from build123d import *

# Parameters (mm, degrees)
SKETCH1_R               = 7.5
BOSS_EXTRUDE2_DEPTH     = 25
CUT_EXTRUDE1_DEPTH      = 24
CUT_EXTRUDE2_DEPTH      = 27
CUT_EXTRUDE2_DEPTH_BACK = 36
SKETCH3_R               = 0.4
SKETCH4_R               = 7
BOSS_EXTRUDE3_DEPTH     = 1
CUT_EXTRUDE3_START      = -11
SKETCH5_R               = 0.4
CUT_EXTRUDE3_DEPTH      = 11


with BuildPart() as part:
    # Sketch1 → Boss-Extrude2 (new body)
    with BuildSketch(Plane.XY):
        with BuildLine():
            ThreePointArc((2.414315168, 0.069999392), (0.769305306, 0.218548989), (-0.013240201, 1.673109733))
            Line((-0.013240201, 1.673109733), (-0.013240201, 23.326890267))
            ThreePointArc((-0.013240201, 23.326890267), (0.497304642, 24.55945455), (1.729868925, 25.069999392))
            Line((1.729868925, 25.069999392), (48.270131075, 25.069999392))
            ThreePointArc((48.270131075, 25.069999392), (49.605427649, 24.447342177), (49.986759799, 23.02421016))
            Line((49.986759799, 23.02421016), (49.986759799, 1.97578984))
            ThreePointArc((49.986759799, 1.97578984), (49.353809753, 0.307800264), (47.585684832, 0.069999392))
            Line((47.585684832, 0.069999392), (2.414315168, 0.069999392))
        make_face()
        with Locations((14.486759799, 15.569999392)):
            Circle(SKETCH1_R, mode=Mode.SUBTRACT)
        with Locations((35.513240201, 15.569999392)):
            Circle(SKETCH1_R, mode=Mode.SUBTRACT)
    extrude(amount=-BOSS_EXTRUDE2_DEPTH)

    # Sketch2 → Cut-Extrude1 (cut)
    with BuildSketch(Plane(origin=(0, 0, -25), x_dir=(-1, 0, 0), z_dir=(0, 0, -1))):
        with BuildLine():
            Line((-0.986759799, 1.673109733), (-0.986759799, 23.326890267))
            ThreePointArc((-0.986759799, 23.326890267), (-1.204411423, 23.852347769), (-1.729868925, 24.069999392))
            Line((-1.729868925, 24.069999392), (-48.270131075, 24.069999392))
            ThreePointArc((-48.270131075, 24.069999392), (-48.861025261, 23.777506771), (-48.986759799, 23.130282932))
            Line((-48.986759799, 23.130282932), (-48.986759799, 1.869717068))
            ThreePointArc((-48.986759799, 1.869717068), (-48.694204694, 1.062886218), (-47.836000807, 1.069999392))
            Line((-47.836000807, 1.069999392), (-2.163999193, 1.069999392))
            ThreePointArc((-2.163999193, 1.069999392), (-1.391043742, 1.011740949), (-0.986759799, 1.673109733))
        make_face()
    extrude(amount=-CUT_EXTRUDE1_DEPTH, mode=Mode.SUBTRACT)

    # Sketch3 → Cut-Extrude2 (cut, two sides: drawn at the far end of the back side and taken through both)
    with BuildSketch(Plane.XZ.offset(-0.069999392).offset(-CUT_EXTRUDE2_DEPTH_BACK)):
        with Locations(Location((25, -12.5, 0), (0, 0, 180))):
            Circle(SKETCH3_R)
    extrude(amount=CUT_EXTRUDE2_DEPTH + CUT_EXTRUDE2_DEPTH_BACK, mode=Mode.SUBTRACT)

    # Sketch4 → Boss-Extrude3 (add)
    with BuildSketch(Plane.XZ.offset(-0.069999392)):
        with Locations((25, -12.5)):
            Circle(SKETCH4_R)
    extrude(amount=BOSS_EXTRUDE3_DEPTH)

    # Sketch5 → Cut-Extrude3 (cut)
    with BuildSketch(Plane(origin=(0, 1.069999392, 0), x_dir=(1, 0, 0), z_dir=(0, 1, 0)).offset(CUT_EXTRUDE3_START)):
        with Locations(Location((25, 12.5, 0), (0, 0, 180))):
            Circle(SKETCH5_R)
    extrude(amount=CUT_EXTRUDE3_DEPTH, mode=Mode.SUBTRACT)


solid = part.part
Read the model definition and answer for the solid it produces. Units are mm, in the model's axes. A direction names the side the tool comes from. Round coordinates to 2 decimals unless told otherwise and drop trailing zeros. Write each loop counter-clockwise with the first axis right and the second up, starting at its lowest first coordinate (ties: lowest second). Pieces come first, ordered by that corner, then holes. Notation, with made-up numbers: (67.25, 58.25) - (121.25, 58.25) arc R10 ccw to (121.25, 71.25) - close; hole circle Ø2 at (-7, 51). An arc over 180 degrees is marked (long way). One line per question, with ' | ' between items. Start each with the question number.
1. Each of these flat-tipped pins is pushed along its axis until it touches: pin 1 (3 mm diameter, centred on x = 44.5, y = 8.5, fed in from -Z); pin 2 (10.5 mm diameter, centred on y = 17.5, z = -7, fed in from +X); pin 3 (2 mm diameter, centred on x = 18, z = -19.5, fed in from -Y); pin 4 (10 mm diameter, centred on x = 34.5, z = -18.5, fed in from -Y). Where does it stop, or does it pass through?
2. Section C-C (x = 33) is taken. Determine the outline of the cut face in (y, z).
3. Find the intervals of material crossed by probe 1 along X at (y, z) = (15.57, -0.45); probe 2 along X at (y, z) = (3.5, -3.5); probe 3 along Y at (x, z) = (12.5, -21.25), in increasing order. Write a range as [from, to].
4. For faces 5 (the face through (0.8, 0.2, -12.3)), 6 (the face through (48.705, 1.07, -13.168)), determine the directions among +Z, -Z, +X, -X, +Y, -Y from which every point of the face is accessible in a straight line to the end or side of a thin tool.
5. Section B-B (y = 10.5) is taken. Determine the outline of the cut face in (x, z).
6. For a pull along X with two mould halves and no side action, classify faces 1 (the face through (-0.013, 12, -12)), 2 (the face through (49.987, 13, -12)), 3 (the face through (24.7, 24.07, -13.2)), 4 (the face through (32.5, 0.5, -25)) as +X half, -X half, draft (parallel to the pull), parting line (faces both ways), or undercut.
7. Section D-D (y = 6.25) is taken. Determine the outline of the cut face in (x, z).
8. Section A-A (z = -22) is taken. Determine the outline of the cut face in (x, y), and give its area (3 significant figures).
Filled in:
1) pin 1: z = -1 | pin 2: x = 49.99 | pin 3: y = 0.07 | pin 4: y = -0.93
2) outline: (0.07, -25) - (1.07, -25) - (1.07, -1) - (8.5, -1) - (8.5, 0) - (0.07, 0) - close; (22.64, -1) - (24.07, -1) - (24.07, -25) - (25.07, -25) - (25.07, 0) - (22.64, 0) - close
3) probe 1: [-0.01, 6.99], [21.99, 28.01], [43.01, 49.99] | probe 2: [-0.01, 0.99], [48.99, 49.99] | probe 3: [0.07, 1.07], [24.07, 25.07]
4) face 5: +Z, -Z, -Y | face 6: -Z
5) outline: (-0.01, -25) - (0.99, -25) - (0.99, -1) - (8.96, -1) - (8.96, 0) - (-0.01, 0) - close; (20.01, -1) - (29.99, -1) - (29.99, 0) - (20.01, 0) - close; (41.04, -1) - (48.99, -1) - (48.99, -25) - (49.99, -25) - (49.99, 0) - (41.04, 0) - close
6) face 1: -X half | face 2: +X half | face 3: undercut | face 4: draft
7) outline: (-0.01, -25) - (0.99, -25) - (0.99, -1) - (48.99, -1) - (48.99, -25) - (49.99, -25) - (49.99, 0) - (-0.01, 0) - close
8) outline: (-0.01, 1.67) arc R1.74 ccw to (2.41, 0.07) - (47.59, 0.07) arc R1.74 ccw to (49.99, 1.98) - (49.99, 23.02) arc R1.74 ccw to (48.27, 25.07) - (1.73, 25.07) arc R1.74 ccw to (-0.01, 23.33) - close; hole (0.99, 1.67) arc R0.74 ccw to (2.16, 1.07) - (47.84, 1.07) arc R0.74 ccw to (48.99, 1.87) - (48.99, 23.13) arc R0.74 ccw to (48.27, 24.07) - (1.73, 24.07) arc R0.74 ccw to (0.99, 23.33) - close | area: 144 mm²
